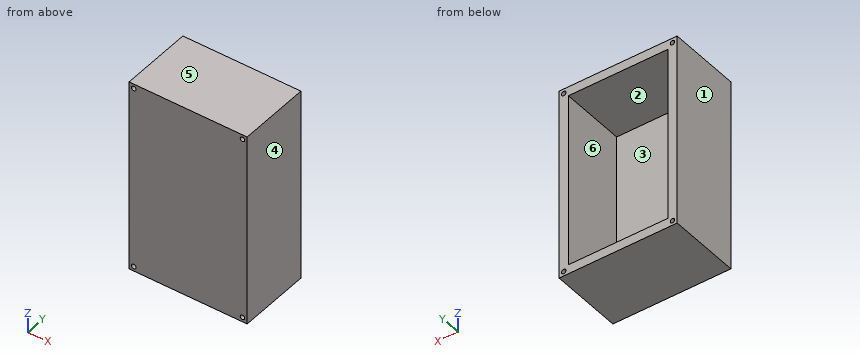
from build123d import *

# Parameters (mm, degrees)
SCHIZZO1_W                   = 63.34
SCHIZZO1_H                   = 103.98
ESTRUSIONE_ESTRUSIONE1_DEPTH = 4
SCHIZZO2_W                   = 63.34
SCHIZZO2_H                   = 103.98
SCHIZZO2_W_2                 = 53.34
SCHIZZO2_H_2                 = 93.98
ESTRUSIONE_ESTRUSIONE2_DEPTH = 35
FORO_PER_VITE_M2_1_D         = 2.4


with BuildPart() as part:
    # Schizzo1 → Estrusione-Estrusione1 (new body)
    with BuildSketch(Plane(origin=(0, 0, 0), x_dir=(1, 0, 0), z_dir=(0, 1, 0))):
        with Locations((34.160538922, 55.414491018)):
            Rectangle(SCHIZZO1_W, SCHIZZO1_H)
    extrude(amount=ESTRUSIONE_ESTRUSIONE1_DEPTH)

    # Schizzo2 → Estrusione-Estrusione2 (add)
    with BuildSketch(Plane(origin=(0, 4, 0), x_dir=(1, 0, 0), z_dir=(0, 1, 0))):
        with Locations((34.160538922, 55.414491018)):
            Rectangle(SCHIZZO2_W, SCHIZZO2_H)
        with Locations((34.160538922, 55.414491018)):
            Rectangle(SCHIZZO2_W_2, SCHIZZO2_H_2, mode=Mode.SUBTRACT)
    extrude(amount=ESTRUSIONE_ESTRUSIONE2_DEPTH)

    # Foro per Vite M2-1 (through all)
    with Locations(Plane(origin=(0, 39, 0), x_dir=(1, 0, 0), z_dir=(0, 1, 0))):
        with Locations((4.990538922, 104.904491018), (63.330538922, 104.904491018), (63.330538922, 5.924491018), (4.990538922, 5.924491018)):
            Hole(FORO_PER_VITE_M2_1_D / 2)


solid = part.part
The model under review builds one solid part; all positions refer to its coordinate system, in mm. Face numbers are marked on the shaded views. A direction names the side the tool comes from. Give positions to 0.01 mm unless a question says otherwise; leave off trailing zeros. Order: outer loops, then holes, each group sorted by start corner. A loop starts at its lowest first (then second) coordinate and runs counter-clockwise, first axis right, second up. Notation, with made-up numbers: M 25,66 L 70,66 A36 cw 70,105 Z; hole C 13,80.25 d4. An arc over 180 degrees is marked long. Answer in a Markdown table with one row per item. Add a question column.
1. To check wall thickness, follow line 1 along Z through (x, y) = (55.5, 8.5); line 2 along X through (y, z) = (10, -90); line 3 along Y through (x, z) = (33.5, -81). State the ranges of each line that lie inside material, in increasing order.
2. For pin 1 Ø10 at (x, z) = (34.5, -88) entering from -Y; pin 2 Ø5 at (x, z) = (49, -57.5) entering from +Y; pin 3 Ø1.4 at (x, z) = (4.99, -104.9) entering from -Y (1 decimal), all flat-tipped, find the tip position at first contact; note any pin that passes through.
3. Add section C-C on y = 16. State the section outline as (x, z) points.
4. Add section A-A on x = 57. State the section outline as (y, z) points.
5. Add section B-B on z = -61.5. State the section outline as (x, y) points, plus the area to 3 significant figures.
6. Machinability: for the marked faces 1 and 2, which of the approach directions +Z, -Z, +X, -X, +Y, -Y give a long, thin tool a straight path to every point of the face, cutting with its end or side? Answer none if there is none.
7. Mouldability with a two-part tool opening along Z and no side actions: class the marked faces 3, 4, 5 and 6 as released by +Z, released by -Z, zero draft, split by the parting line, or undercut.
The answers:
| question | item | result |
|---|---|---|
| 1 | line 1 | -107.4 to -102.4, -8.42 to -3.42 |
| 1 | line 2 | 2.49 to 7.49, 60.83 to 65.83 |
| 1 | line 3 | 0 to 4 |
| 2 | pin 1 | y = 0 |
| 2 | pin 2 | y = 4 |
| 2 | pin 3 | through |
| 3 | outline | M 2.49,-107.4 L 65.83,-107.4 L 65.83,-3.42 L 2.49,-3.42 Z; hole C 4.99,-104.9 d2.4; hole C 4.99,-5.92 d2.4; hole M 7.49,-102.4 L 60.83,-102.4 L 60.83,-8.42 L 7.49,-8.42 Z; hole C 63.33,-104.9 d2.4; hole C 63.33,-5.92 d2.4 |
| 4 | outline | M 0,-107.4 L 39,-107.4 L 39,-102.4 L 4,-102.4 L 4,-8.42 L 39,-8.42 L 39,-3.42 L 0,-3.42 Z |
| 5 | outline | M 2.49,0 L 65.83,0 L 65.83,39 L 60.83,39 L 60.83,4 L 7.49,4 L 7.49,39 L 2.49,39 Z |
| 5 | area | 603 mm2 |
| 6 | face 1 | +Z, -Z, -X, +Y, -Y |
| 6 | face 2 | +Y |
| 7 | face 3 | undercut |
| 7 | face 4 | zero draft |
| 7 | face 5 | released by +Z |
| 7 | face 6 | undercut |
